Autodesk Inventor part; units mm, degrees
ref_plane "YZ Plane" through (0, 0, 0) normal (1, 0, 0) x (0, 1, 0)
ref_plane "XZ Plane" through (0, 0, 0) normal (0, 1, 0) x (-1, 0, 0)
ref_plane "XY Plane" through (0, 0, 0) normal (0, 0, 1) x (1, 0, 0)
sketch "Sketch1" plane through (0, 0, 0) normal (0, 0, 1) x (1, 0, 0)
  line L0 (-63.5, -20) -> (63.5, -20)
  line L1 (63.5, -20) -> (63.5, 20)
  line L2 (63.5, 20) -> (-63.5, 20)
  line L3 (-63.5, 20) -> (-63.5, -20)
  line L4 (-63.5, -20) -> (63.5, 20) construction
  line L5 (63.5, -20) -> (-63.5, 20) construction
  line L6 (-63.5, 9) -> (-60.5, 9)
  line L7 (-60.5, 9) -> (-60.5, -6) construction
  line L8 (-60.5, -6) -> (-63.5, -6)
  line L9 (-63.5, -6) -> (-63.5, 9)
  line L10 (-63.5, 9) -> (-60.5, -6) construction
  line L11 (-60.5, 9) -> (-63.5, -6) construction
  line L12 (-45.1, 20) -> (-24.9, 20)
  line L13 (-24.9, 20) -> (-24.9, 17)
  line L14 (-24.9, 17) -> (-45.1, 17)
  line L15 (-45.1, 17) -> (-45.1, 20)
  line L16 (-45.1, 20) -> (-24.9, 17) construction
  line L17 (-24.9, 20) -> (-45.1, 17) construction
  line L18 (-10.1, 20) -> (10.1, 20)
  line L19 (10.1, 20) -> (10.1, 17)
  line L20 (10.1, 17) -> (-10.1, 17)
  line L21 (-10.1, 17) -> (-10.1, 20)
  line L22 (-10.1, 20) -> (10.1, 17) construction
  line L23 (10.1, 20) -> (-10.1, 17) construction
  line L24 (24.9, 20) -> (45.1, 20)
  line L25 (45.1, 20) -> (45.1, 17)
  line L26 (45.1, 17) -> (24.9, 17)
  line L27 (24.9, 17) -> (24.9, 20)
  line L28 (24.9, 20) -> (45.1, 17) construction
  line L29 (45.1, 20) -> (24.9, 17) construction
  line L30 (-60.5, 9) -> (-60.5, 20)
  line L31 (-60.5, -6) -> (-60.5, -20)
  point P0 (0, 0)
  point P1 (-62, 1.5)
  point P2 (-63.5, 0)
  point P3 (-35, 18.5)
  point P4 (0, 18.5)
  point P5 (35, 18.5)
  point P6 (0, 20)
  point P7 (45.1, 20)
  point P8 (24.9, 20)
  point P9 (10.1, 20)
  point P10 (-45.1, 20)
  dimension "d0" = 127
  dimension "d1" = 40
  dimension "d2" = 3
  dimension "d3" = 15
  dimension "d4" = 20.2
  dimension "d5" = 3
  dimension "d6" = 20.2
  dimension "d7" = 3
  dimension "d8" = 20.2
  dimension "d9" = 3
  dimension "d10" = 35
  dimension "d11" = 35
  dimension "d16" = 1.5
extrude "Extrusion1" add sketch "Sketch1" along normal blind 3 contours L3 L8 L31 L0 | L31 L8 L3 L6 L30 L2 L15 L14 L13 L21 L20 L19 L27 L26 L25 L1 L0 | L3 L2 L30 L6
extrude "Extrusion2" cut sketch "Sketch1" along normal through all contours L3 L8 L31 L0 | L3 L2 L30 L6 | L25 L26 L27 L2 | L2 L13 L14 L15 | L19 L20 L21 L2
mirror "Mirror1" about plane through (0, 0, 0) normal (1, 0, 0) of "Extrusion2"
equation "\"d5\" = d2"
equation "\"d6\" = d4"
equation "\"d7\" = d5"
equation "\"d8\" = d6"
equation "\"d9\" = d7"
properties part number "bed_acrylic_upper_floort"
Read the model definition and answer for the solid it produces. Units are mm, in the model's axes. A direction names the side the tool comes from. Coordinates: 2 decimals unless noted, no trailing zeros. Write each loop counter-clockwise with the first axis right and the second up, starting at its lowest first coordinate (ties: lowest second). Pieces come first, ordered by that corner, then holes. Notation, with made-up numbers: (75.25, 60) -> (109.25, 60) arc R32 ccw to (109.25, 92) -> close; hole circle Ø11 at (21, 50.25). An arc over 180 degrees is marked (long way). Return JSON: item names as keys, results as strings.
(1) Each of these flat-tipped pins is pushed along its axis until it touches: P1, Ø1.5, axis at x = 39, z = 1, coming from the +Y side; P2, Ø0.9, axis at y = 19, z = 1, coming from the -X side; P3, Ø0.9, axis at x = 62, z = 1, coming from the +Y side. Where does it stop, or does it pass through?
Answers below:
{"P1": "y = 17", "P2": "x = -60.5", "P3": "y = 9"}
(2) The part is cut by section C-C on y = -15. Give the vertices of the cut face in (x, z).
Answers below:
{"outline": "(-60.5, 0) -> (60.5, 0) -> (60.5, 3) -> (-60.5, 3) -> close"}
(3) The part is cut by section B-B on x = 42. Give the vertices of the cut face in (y, z), then the cut area to 3 significant figures.
Answers below:
{"outline": "(-20, 0) -> (17, 0) -> (17, 3) -> (-20, 3) -> close", "area": "111 mm^2"}
(4) The part is cut by section A-A on z = 0.45. Give the vertices of the cut face in (x, y), then the cut area to 3 significant figures.
Answers below:
{"outline": "(-63.5, -6) -> (-60.5, -6) -> (-60.5, -20) -> (60.5, -20) -> (60.5, -6) -> (63.5, -6) -> (63.5, 9) -> (60.5, 9) -> (60.5, 20) -> (45.1, 20) -> (45.1, 17) -> (24.9, 17) -> (24.9, 20) -> (10.1, 20) -> (10.1, 17) -> (-10.1, 17) -> (-10.1, 20) -> (-24.9, 20) -> (-24.9, 17) -> (-45.1, 17) -> (-45.1, 20) -> (-60.5, 20) -> (-60.5, 9) -> (-63.5, 9) -> close", "area": "4,750 mm^2"}
(5) Which of the six approach directions +Z, -Z, +X, -X, +Y, -Y give full straight-line access (tool end or side, diameter ignored) to faces 5 (the flat face through (45.1, 19, 1)), 6 (the flat face through (60.5, 15, 1)), 7 (the flat face through (60.5, -13, 1))?
Answers below:
{"face 5": "+Z, -Z, +Y", "face 6": "+Z, -Z, +X, +Y", "face 7": "+Z, -Z, +X, -Y"}
(6) For a pull along X with two mould halves and no side action, classify faces 1 (the flat face through (53, 20, 1)), 2 (the flat face through (10.1, 19, 1)), 3 (the flat face through (-63.5, 2, 1)), 4 (the flat face through (63.5, 1, 1)) as pulls with the +X half, pulls with the -X half, needs draft (parallel to the pull), parting line crosses it, or undercut.
Answers below:
{"face 1": "needs draft", "face 2": "undercut", "face 3": "pulls with the -X half", "face 4": "pulls with the +X half"}
(7) Consider line 1 along X through (y, z) = (18.5, 2.6); line 2 along Y through (x, z) = (43, 1.1); line 3 along X through (y, z) = (-14, 0.2). Determine where each line is inside the solid, lowest interval first. Write a range as from..to.
Answers below:
{"line 1": "-60.5..-45.1, -24.9..-10.1, 10.1..24.9, 45.1..60.5", "line 2": "-20..17", "line 3": "-60.5..60.5"}
